```python
from build123d import *
from build123d.topology import SkipClean

# Parameters (mm, degrees)
SKETCH1_R           = 19.05
BOSS_EXTRUDE1_DEPTH = 19.558
SKETCH2_R           = 6.35
BOSS_EXTRUDE2_DEPTH = 60.96
SKETCH3_R           = 19.05
BOSS_EXTRUDE3_DEPTH = 6.35


with BuildPart() as part:
    # Sketch1 → Boss-Extrude1 (new body)
    with BuildSketch(Plane(origin=(0, 0, 0), x_dir=(0, 0, -1), z_dir=(1, 0, 0))):
        with BuildLine():
            Line((25.4, 62.611), (-25.4, 62.611))
            ThreePointArc((-25.4, 62.611), (-43.71389723, 59.350669702), (-59.777434529, 49.970298982))
            Line((-59.777434529, 49.970298982), (-101.281034529, 14.478))
            ThreePointArc((-101.281034529, 14.478), (-80.929937509, 17.302618411), (-69.85, 0))
            ThreePointArc((-69.85, 0), (-80.929937509, -17.302618411), (-101.281034529, -14.478))
            Line((-101.281034529, -14.478), (-59.777434529, -49.970298982))
            ThreePointArc((-59.777434529, -49.970298982), (-43.71389723, -59.350669702), (-25.4, -62.611))
            Line((-25.4, -62.611), (25.4, -62.611))
            ThreePointArc((25.4, -62.611), (43.699078076, -59.34404997), (59.737214243, -49.946847768))
            Line((59.737214243, -49.946847768), (101.269374674, -14.487973703))
            ThreePointArc((101.269374674, -14.487973703), (69.85, -7.706e-06), (101.269379322, 14.48794821))
            Line((101.269379322, 14.48794821), (59.737230268, 49.9468356))
            ThreePointArc((59.737230268, 49.9468356), (43.699087699, 59.344046737), (25.4, 62.611))
        make_face()
        with Locations((88.9, -1.0762e-05)):
            Circle(SKETCH1_R)
        with Locations((-88.9, 0)):
            Circle(SKETCH1_R)
    extrude(amount=BOSS_EXTRUDE1_DEPTH)

    # Sketch2 → Boss-Extrude2 (add)
    with BuildSketch(Plane(origin=(19.558, 0, 0), x_dir=(0, 0, -1), z_dir=(1, 0, 0))):
        with Locations(Location((-88.9, 0, 0), (0, 0, 180))):
            Circle(SKETCH2_R)
        with Locations(Location((88.9, -1.0762e-05, 0), (0, 0, 180))):
            Circle(SKETCH2_R)
    extrude(amount=BOSS_EXTRUDE2_DEPTH)

    # Sketch3 → Boss-Extrude3 (add)
    with SkipClean():  # the faces are left unmerged after this step: merging them gives an invalid solid
        with BuildSketch(Plane(origin=(19.558, 0, 0), x_dir=(0, 0, -1), z_dir=(1, 0, 0))):
            with Locations(Location((-88.9, 0, 0), (0, 0, 130.535802111))):
                Circle(SKETCH3_R)
            with Locations(Location((88.9, -1.0762e-05, 0), (0, 0, 310.489674839))):
                Circle(SKETCH3_R)
        extrude(amount=BOSS_EXTRUDE3_DEPTH)


solid = part.part
```
Design review of the part built by this model. Coordinates are the model's own, in mm. A direction names the side the tool comes from. Coordinates: 2 decimals unless noted, no trailing zeros. Write each loop counter-clockwise with the first axis right and the second up, starting at its lowest first coordinate (ties: lowest second). Pieces come first, ordered by that corner, then holes. Notation, with made-up numbers: M 69.5,-2.5 L 93.5,-2.5 A10 cw 93.5,16.5 Z; hole C -7.5,57.25 d9. An arc over 180 degrees is marked long. Answer as a JSON object with one key per item and string values.
Item 1: Draft analysis for pull direction Z (two halves, no side actions). For faces 3 (the flat face through (25.908, 5, 82)), 4 (the flat face through (80.518, 0, 89)), 5 (the cylindrical face through (9.642, 59.253, -43.944)), 6 (the flat face through (25.908, -5, -82)), state which applies: pulls with the +Z half, pulls with the -Z half, needs draft (parallel to the pull), parting line crosses it, or undercut.
Outcome:
{"face 3": "undercut", "face 4": "needs draft", "face 5": "pulls with the -Z half", "face 6": "undercut"}
Item 2: Machinability: for faces 1 (the cylindrical face through (9.642, -59.434, -43.453)), 2 (the cylindrical face through (52.831, -1.907, -82.843)), which of the approach directions +Z, -Z, +X, -X, +Y, -Y give a long, thin tool a straight path to every point of the face, cutting with its end or side? Answer none if there is none.
Outcome:
{"face 1": "-Z, +X, -X, -Y", "face 2": "+X"}
Item 3: Add section B-B, the plane x = 50. Give the boundary of the cut face in (y, z), and give its area (3 significant figures).
Outcome:
{"outline": "C 0,-88.9 d12.7; C 0,88.9 d12.7", "area": "253 mm²"}
Item 4: Add section C-C, the plane y = -42. Give the boundary of the cut face in (x, z).
Outcome:
{"outline": "M 0,-69.05 L 19.56,-69.05 L 19.56,69.1 L 0,69.1 Z"}
Item 5: Add section D-D, the plane z = 88.9. Give the boundary of the cut face in (x, y).
Outcome:
{"outline": "M 0,-25.07 L 19.56,-25.07 L 19.56,-19.05 L 25.91,-19.05 L 25.91,-6.35 L 80.52,-6.35 L 80.52,6.35 L 25.91,6.35 L 25.91,19.05 L 19.56,19.05 L 19.56,25.07 L 0,25.07 Z"}
Item 6: Add section A-A, the plane z = -92. Give the boundary of the cut face in (x, y).
Outcome:
{"outline": "M 0,-22.4 L 19.56,-22.4 L 19.56,-18.8 L 25.91,-18.8 L 25.91,-5.54 L 80.52,-5.54 L 80.52,5.54 L 25.91,5.54 L 25.91,18.8 L 19.56,18.8 L 19.56,22.4 L 0,22.4 Z"}
Item 7: Wall thickness on probe 1 along X at (y, z) = (-10, -66.5); probe 2 along Z at (x, y) = (24, -16.5); probe 3 along Y at (x, z) = (15, 31): over which ranges is each line inside the solid? List them lowest first.
Outcome:
{"probe 1": "0 to 19.56", "probe 2": "-98.42 to -79.38, 79.38 to 98.42", "probe 3": "-62.31 to 62.31"}
Item 8: Insertion check: pin 1 Ø6 at (y, z) = (48.5, -31) entering from +X. The pin has a flat end and moves straight along its axis. Give the tip position at first contact, or say it passes through.
Outcome:
{"pin 1": "x = 19.56"}
